Part print with two shaded views. Sizes in mm from the minimum x, y, z corner. A direction names the side the tool comes from. Give positions to 0.01 mm unless a question says otherwise; leave off trailing zeros. Write each loop counter-clockwise with the first axis right and the second up, starting at its lowest first coordinate (ties: lowest second). Pieces come first, ordered by that corner, then holes.
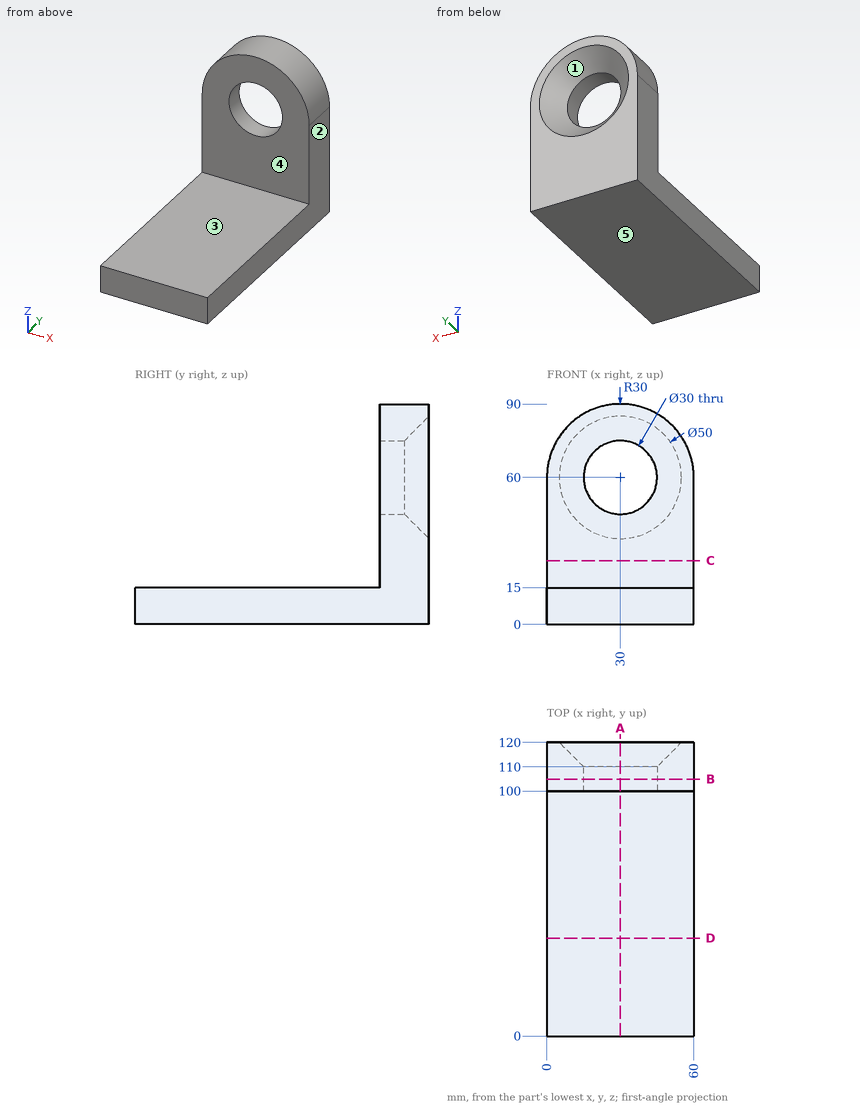
1) Pin check, flat tips, straight feed: pin 1 Ø18 at (x, y) = (34, 32.5) entering from +Z; pin 2 Ø10 at (x, y) = (43, 22) entering from -Z; pin 3 Ø10 at (x, z) = (38, 80) entering from -Y. Stop position of each tip, or through.
Answers follow:
pin 1: stops at z = 15
pin 2: stops at z = 0
pin 3: stops at y = 100
2) Two-plate mould, pull along X, no slides. Class the marked faces 1, 2 and 3: +X half, -X half, draft (parallel to the pull), parting line (faces both ways), or undercut.
Answers follow:
face 1: undercut
face 2: +X half
face 3: draft
3) Saw through at D-D, the plane y = 40. Write the cut outline in (x, z), then the cut area to 3 significant figures.
Answers follow:
outline: (0, 0) - (60, 0) - (60, 15) - (0, 15) - close
area: 900 mm2
4) Wall check: L1, parallel to Z at x = 30, y = 104; L2, parallel to Z at x = 50, y = 67.5; L3, parallel to Y at x = 55, z = 76.5. Give the ranges that are in metal, low to high.
Answers follow:
L1: z = 0 to 45, 75 to 90
L2: z = 0 to 15
L3: y = 100 to 120
5) Saw through at A-A, the plane x = 30. Write the cut outline in (y, z), then the cut area to 3 significant figures.
Answers follow:
outline: (0, 0) - (120, 0) - (120, 35) - (110, 45) - (100, 45) - (100, 15) - (0, 15) - close; (100, 75) - (110, 75) - (120, 85) - (120, 90) - (100, 90) - close
area: 2,600 mm2
6) 3-axis set-ups, long thin cutter, end or side, ignore diameter. For the marked faces 4 and 5: which of +Z, -Z, +X, -X, +Y, -Y reach the whole face in a straight line?
Answers follow:
face 4: +Z, +X, -X, -Y
face 5: -Z, +X, -X, +Y, -Y
7) Saw through at C-C, the plane z = 26. Write the cut outline in (x, y), then the cut area to 3 significant figures.
Answers follow:
outline: (0, 100) - (60, 100) - (60, 120) - (0, 120) - close
area: 1,200 mm2
8) Saw through at B-B, the plane y = 105. Write the cut outline in (x, z), then the cut area to 3 significant figures.
Answers follow:
outline: (0, 0) - (60, 0) - (60, 60) arc R30 ccw to (0, 60) - close; hole circle Ø30 at (30, 60)
area: 4,310 mm2
